Build history of the part. All positions in model axes, mm. A direction names the side the tool comes from. Round coordinates to 2 decimals unless told otherwise and drop trailing zeros. Write each loop counter-clockwise with the first axis right and the second up, starting at its lowest first coordinate (ties: lowest second). Pieces come first, ordered by that corner, then holes. Notation, with made-up numbers: M 13.5,39.5 L 52.5,39.5 A18 ccw 52.5,46.5 Z; hole C -7,77.5 d11. An arc over 180 degrees is marked long. Use a Markdown table: item, result.
from build123d import *

# Parameters (mm, degrees)
SKETCH1_R           = 3.5
BOSS_EXTRUDE1_DEPTH = 87.927
SKETCH2_R           = 1.75
CUT_EXTRUDE1_DEPTH  = 8.9
CUT_EXTRUDE2_START  = -87.927
SKETCH2_2_R         = 1.75
CUT_EXTRUDE2_DEPTH  = 8.9
CUT_EXTRUDE3_REACH  = 9
SKETCH3_R           = 1.75
BOSS_EXTRUDE2_DEPTH = 7.5
SKETCH5_R           = 1.5
SKETCH5_R_2         = 3.5
BOSS_EXTRUDE3_DEPTH = 5.2
SKETCH6_R           = 3.5
SKETCH6_R_2         = 1.75
BOSS_EXTRUDE5_DEPTH = 1.1
SKETCH7_R           = 1.75
BOSS_EXTRUDE6_DEPTH = 0.4
SKETCH8_R           = 1.75
BOSS_EXTRUDE7_DEPTH = 1.473


with BuildPart() as part:
    # Sketch1 → Boss-Extrude1 (new body)
    with BuildSketch(Plane(origin=(0, 0, 0), x_dir=(1, 0, 0), z_dir=(0, 1, 0))):
        Circle(SKETCH1_R)
    extrude(amount=BOSS_EXTRUDE1_DEPTH)

    # Sketch2 → Cut-Extrude1 (cut)
    with BuildSketch(Plane.XZ):
        Circle(SKETCH2_R)
    extrude(amount=-CUT_EXTRUDE1_DEPTH, mode=Mode.SUBTRACT)

    # Sketch2<2> → Cut-Extrude2 (cut)
    with BuildSketch(Plane.XZ.offset(CUT_EXTRUDE2_START)):
        Circle(SKETCH2_2_R)
    extrude(amount=CUT_EXTRUDE2_DEPTH, mode=Mode.SUBTRACT)

    # Sketch3 → Cut-Extrude3 (cut, up to next)
    with BuildSketch(Plane.ZY.offset(3.5), mode=Mode.PRIVATE) as cut_extrude3_sk1:
        with Locations((0, 4.677)):
            Circle(SKETCH3_R)
    cut_extrude3_tool1 = extrude(cut_extrude3_sk1.sketch, amount=-CUT_EXTRUDE3_REACH, mode=Mode.PRIVATE) & part.part
    add(cut_extrude3_tool1.solids().sort_by_distance((-3.5, 4.677, 0))[0], mode=Mode.SUBTRACT)
    # Sketch3 → Cut-Extrude3 (cut, up to next)
    with BuildSketch(Plane.ZY.offset(3.5), mode=Mode.PRIVATE) as cut_extrude3_sk2:
        with Locations((0, 82.177)):
            Circle(SKETCH3_R)
    cut_extrude3_tool2 = extrude(cut_extrude3_sk2.sketch, amount=-CUT_EXTRUDE3_REACH, mode=Mode.PRIVATE) & part.part
    add(cut_extrude3_tool2.solids().sort_by_distance((-3.5, 82.177, 0))[0], mode=Mode.SUBTRACT)

    # Sketch4 → Boss-Extrude2 (add)
    with BuildSketch(Plane(origin=(0, 68.677, 0), x_dir=(1, 0, 0), z_dir=(0, 1, 0))):
        with BuildLine():
            Line((0.85, 3.240370349), (0.85, 4.704101966))
            Line((0.85, 4.704101966), (-0.85, 4.704101966))
            Line((-0.85, 4.704101966), (-0.85, 3.240370349))
            ThreePointArc((-0.85, 3.240370349), (0, -3.35), (0.85, 3.240370349))
        make_face()
    extrude(amount=-BOSS_EXTRUDE2_DEPTH)

    # Sketch5 → Boss-Extrude3 (add)
    with BuildSketch(Plane.XZ.offset(-61.177)):
        with BuildLine():
            Line((-3.944053189, 0.666666667), (-2.465033243, 9.416666667))
            ThreePointArc((-2.465033243, 9.416666667), (0, 11.5), (2.465033243, 9.416666667))
            Line((2.465033243, 9.416666667), (3.944053189, 0.666666667))
            ThreePointArc((3.944053189, 0.666666667), (4, 0), (3.944053189, -0.666666667))
            Line((3.944053189, -0.666666667), (2.465033243, -9.416666667))
            ThreePointArc((2.465033243, -9.416666667), (0, -11.5), (-2.465033243, -9.416666667))
            Line((-2.465033243, -9.416666667), (-3.944053189, -0.666666667))
            ThreePointArc((-3.944053189, -0.666666667), (-4, 0), (-3.944053189, 0.666666667))
        make_face()
        with Locations((0, 9)):
            Circle(SKETCH5_R, mode=Mode.SUBTRACT)
        Circle(SKETCH5_R_2, mode=Mode.SUBTRACT)
        with Locations((0, -9)):
            Circle(SKETCH5_R, mode=Mode.SUBTRACT)
    extrude(amount=BOSS_EXTRUDE3_DEPTH)

    # Sketch6 → Boss-Extrude5 (add)
    with BuildSketch(Plane(origin=(0, 0, 0), x_dir=(1, 0, 0), z_dir=(0, 1, 0))):
        Circle(SKETCH6_R)
        Circle(SKETCH6_R_2, mode=Mode.SUBTRACT)
    extrude(amount=-BOSS_EXTRUDE5_DEPTH)

    # Sketch7 → Boss-Extrude6 (add)
    with BuildSketch(Plane(origin=(0, 79.027, 0), x_dir=(1, 0, 0), z_dir=(0, 1, 0))):
        Circle(SKETCH7_R)
    extrude(amount=BOSS_EXTRUDE6_DEPTH)

    # Sketch8 → Boss-Extrude7 (add)
    with BuildSketch(Plane.XZ.offset(-8.9)):
        Circle(SKETCH8_R)
    extrude(amount=BOSS_EXTRUDE7_DEPTH)


solid = part.part
Q1. Two-plate mould, pull along X, no slides. Class faces 1 (the flat face through (0, 79.427, 0)), 2 (the flat face through (3.215, 58.613, -4.98)), 3 (the cylindrical face through (0, 58.6, -11.5)): +X half, -X half, draft (parallel to the pull), parting line (faces both ways), or undercut.
Response values:
| item | result |
|---|---|
| face 1 | undercut |
| face 2 | +X half |
| face 3 | parting line |
Q2. Which spindle directions (+Z, -Z, +X, -X, +Y, -Y) get a long thin tool onto all of the face, cutting with end or side? Do faces 4 (the cylindrical face through (-2.16, 6.41, -0.23)), 5 (the flat face through (0, 7.427, 0)), 6 (the flat face through (0, 65, -4.704)), 7 (the cylindrical face through (1.669, 83.736, 0.526)). Say none if no direction does.
Response values:
| item | result |
|---|---|
| face 4 | -X |
| face 5 | -Y |
| face 6 | -Z, +X, -X, +Y |
| face 7 | +Y |
Q3. Cut at A-A on y = 57.5. Give the cut face in (x, z), and give its area (3 significant figures).
Response values:
| item | result |
|---|---|
| outline | M -3.94,-0.67 L -2.47,-9.42 A2.5 ccw 2.47,-9.42 L 3.94,-0.67 A4 ccw 3.94,0.67 L 2.47,9.42 A2.5 ccw -2.47,9.42 L -3.94,0.67 A4 ccw Z; hole C 0,-9 d3; hole C 0,9 d3 |
| area | 124 mm2 |
Q4. Cut at C-C on y = 13. Give the cut face in (x, z).
Response values:
| item | result |
|---|---|
| outline | C 0,0 d7 |
Q5. Cut at B-B on z = 8.25. Give the cut face in (x, y).
Response values:
| item | result |
|---|---|
| outline | M -2.66,55.98 L -1.3,55.98 L -1.3,61.18 L -2.66,61.18 Z; M 1.3,55.98 L 2.66,55.98 L 2.66,61.18 L 1.3,61.18 Z |
Q6. Drill centre lines: L1, parallel to Z at x = 0, y = 86.25; L2, parallel to Z at x = 0, y = 55; L3, parallel to Y at x = 0, z = -5. Where is each one in solid material? Low to high.
Response values:
| item | result |
|---|---|
| L1 | z = -3.5 to -1.75, 1.75 to 3.5 |
| L2 | z = -3.5 to 3.5 |
| L3 | y = 55.98 to 61.18 |
Q7. Drop flat-ended pins along their axis: P1, Ø3.5, axis at x = 0, z = 9, coming from the +Y side; P2, Ø1.8, axis at x = -0.5, z = 0, coming from the -Y side; P3, Ø4, axis at x = -1, y = 75, coming from the -Z side. Give the stop position or say it passes through.
Response values:
| item | result |
|---|---|
| P1 | stops at y = 61.18 |
| P2 | stops at y = 7.43 |
| P3 | stops at z = -3.5 |
